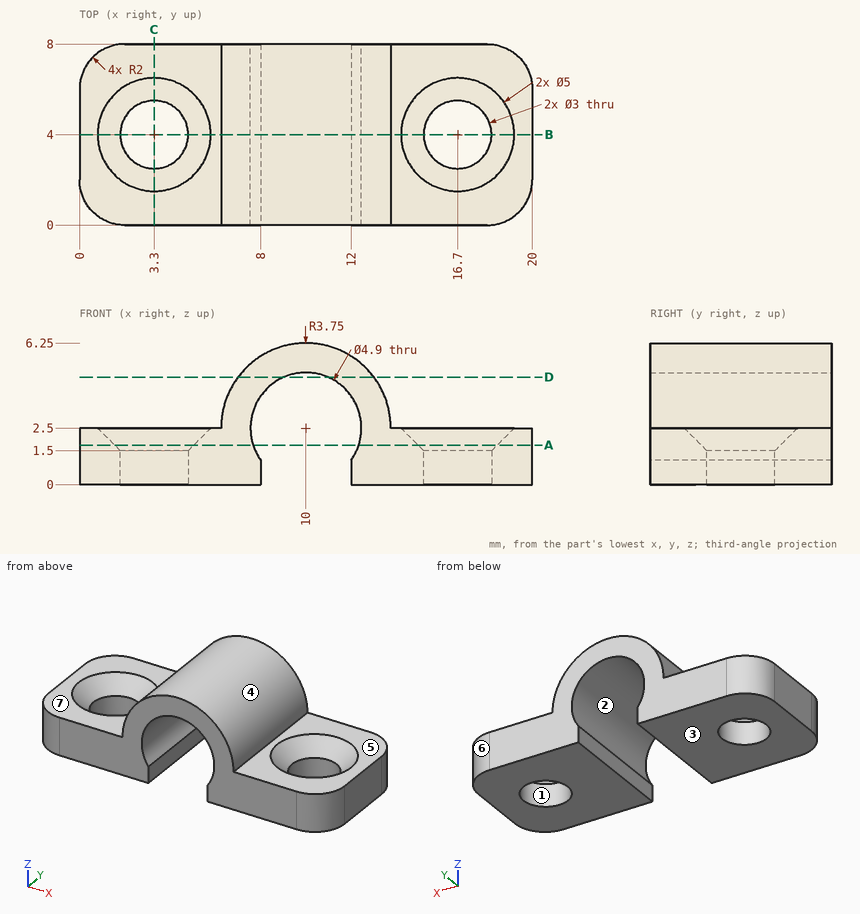
Check sheet for the drawn part. Datum: minimum x, y, z corner. Units: mm. A direction names the side the tool comes from. Round coordinates to 2 decimals unless told otherwise and drop trailing zeros. Order: outer loops, then holes, each group sorted by start corner. A loop starts at its lowest first (then second) coordinate and runs counter-clockwise, first axis right, second up. Notation, with made-up numbers: (-13, 36) -> (4, 36) arc R10 ccw to (4, 44) -> close; hole circle Ø5 at (61, 65.5). An arc over 180 degrees is marked (long way). Put each result on its own line as item: value. Start each with the question number.
(1) Depth check by flat-ended pin: pin 1 Ø1.5 at (y, z) = (1, 1.5) entering from -X; pin 2 Ø1.9 at (x, y) = (2.5, 2) entering from +Z. Enter the tip coordinate at first touch or a pass-through.
(2) Material ranges on line 1 along Y through (x, z) = (16.7, 1.25); line 2 along X through (y, z) = (3.75, 2); line 3 along Z through (x, y) = (6, 6.5), recorded low to high.
(3) Section check C-C (x = 3.3). Enter the section's corners in (y, z).
(4) Draft check along Z on the marked faces 1, 2, 3 and 4. Enter one of: +Z half, -Z half, draft (parallel to the pull), parting line (faces both ways), or undercut.
(5) Section check D-D (z = 4.75). Enter the section's corners in (x, y).
(6) Tool access check on the marked faces 5, 6 and 7. Record the directions out of +Z, -Z, +X, -X, +Y, -Y that give a thin tool (end or side, any length) a straight path to the whole face; none if there is none.
(7) Section check B-B (y = 4). Enter the section's corners in (x, z), then the cut area to 3 significant figures.
(8) Section check A-A (z = 1.75). Enter the section's corners in (x, y).
Completed:
1. pin 1: stops at x = 0.02
1. pin 2: stops at z = 2.5
2. line 1: y = 0 to 2.5, 5.5 to 8
2. line 2: x = 0 to 1.32, 5.28 to 7.6, 12.4 to 14.72, 18.68 to 20
2. line 3: z = 0 to 2.5
3. outline: (0, 0) -> (2.5, 0) -> (2.5, 1.5) -> (1.5, 2.5) -> (0, 2.5) -> close; (5.5, 0) -> (8, 0) -> (8, 2.5) -> (6.5, 2.5) -> (5.5, 1.5) -> close
4. face 1: draft
4. face 2: undercut
4. face 3: -Z half
4. face 4: +Z half
5. outline: (7, 0) -> (9.03, 0) -> (9.03, 8) -> (7, 8) -> close; (10.97, 0) -> (13, 0) -> (13, 8) -> (10.97, 8) -> close
6. face 5: +Z, +X, +Y, -Y
6. face 6: +Z, -Z, +X, +Y
6. face 7: +Z, -X, +Y, -Y
7. outline: (0, 0) -> (1.8, 0) -> (1.8, 1.5) -> (0.8, 2.5) -> (0, 2.5) -> close; (4.8, 0) -> (8, 0) -> (8, 1.08) arc R2.45 cw (long way) to (12, 1.08) -> (12, 0) -> (15.2, 0) -> (15.2, 1.5) -> (14.2, 2.5) -> (13.75, 2.5) arc R3.75 ccw to (6.25, 2.5) -> (5.8, 2.5) -> (4.8, 1.5) -> close; (18.2, 0) -> (20, 0) -> (20, 2.5) -> (19.2, 2.5) -> (18.2, 1.5) -> close
7. area: 34.8 mm2
8. outline: (0, 2) arc R2 ccw to (2, 0) -> (7.67, 0) -> (7.67, 8) -> (2, 8) arc R2 ccw to (0, 6) -> close; (12.33, 0) -> (18, 0) arc R2 ccw to (20, 2) -> (20, 6) arc R2 ccw to (18, 8) -> (12.33, 8) -> close; hole circle Ø3.5 at (3.3, 4); hole circle Ø3.5 at (16.7, 4)
